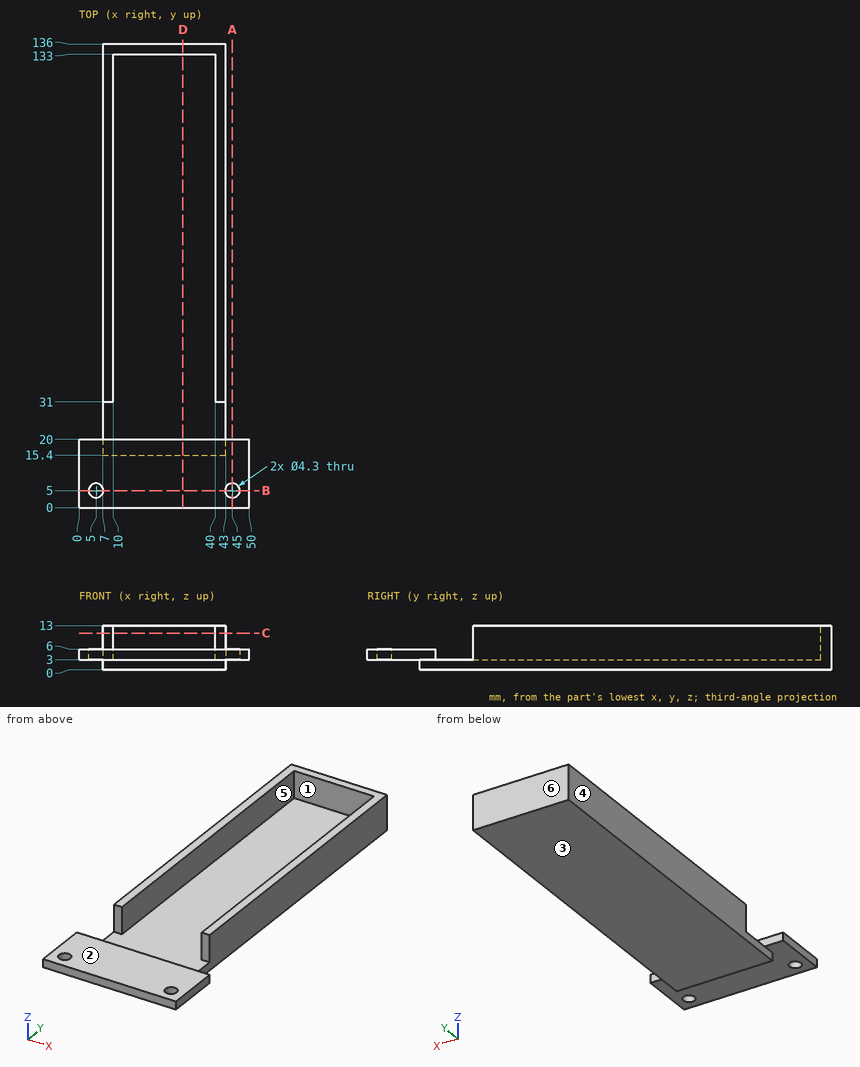
The drawing under review shows one solid part. Ordinate dimensions are in mm from its lowest x, y, z. A direction names the side the tool comes from. Round coordinates to 2 decimals unless told otherwise and drop trailing zeros. Loops run counter-clockwise (first coordinate to the right, second up) from the corner with the lowest first, then second, coordinate; pieces in that order, holes last. Notation, with made-up numbers: (45.25, 76) - (63.25, 76) arc R18 cw to (63.25, 83) - close; hole circle Ø5 at (32.25, 1.25). An arc over 180 degrees is marked (long way). Use a Markdown table: item, result. Add a question column.
Q1. Add section D-D (x = 30.5). State the section outline as (y, z) points, plus the area to 3 significant figures.
Q2. The part is to be moulded in two halves that separate along Y. For the marked faces 4, 5 and 6, say which applies: pulls with the +Y half, pulls with the -Y half, needs draft (parallel to the pull), parting line crosses it, or undercut.
Q3. Insertion check: pin 1 Ø5.5 at (x, y) = (5, 5) entering from +Z; pin 2 Ø1 at (y, z) = (109.5, 7.5) entering from -X; pin 3 Ø3.5 at (x, y) = (45, 5) entering from +Z; pin 4 Ø1.5 at (x, z) = (31, 1.5) entering from -Y. Each pin has a flat end and moves straight along its axis. Give the tip position at first contact, or say it passes through.
Q4. Add section C-C (z = 10.75). State the section outline as (x, y) points.
Q5. Machinability: for the marked faces 1, 2 and 3, which of the approach directions +Z, -Z, +X, -X, +Y, -Y give a long, thin tool a straight path to every point of the face, cutting with its end or side? Answer none if there is none.
Q6. Add section A-A (x = 45). State the section outline as (y, z) points.
Q7. Add section B-B (y = 5). State the section outline as (x, z) points.
Q8. For probe 1 along Y at (x, z) = (45, 4.3); probe 2 along X at (y, z) = (110.5, 8); probe 3 along Y at (x, z) = (35, 3.75), list the stretches that pass through material, from the lowest coordinate up.
Worked answers:
| question | item | result |
|---|---|---|
| 1 | outline | (0, 3) - (15.4, 3) - (15.4, 0) - (136, 0) - (136, 13) - (133, 13) - (133, 3) - (20, 3) - (20, 6) - (0, 6) - close |
| 1 | area | 452 mm² |
| 2 | face 4 | needs draft |
| 2 | face 5 | undercut |
| 2 | face 6 | pulls with the +Y half |
| 3 | pin 1 | z = 6 |
| 3 | pin 2 | x = 7 |
| 3 | pin 3 | through |
| 3 | pin 4 | y = 15.4 |
| 4 | outline | (7, 31) - (10, 31) - (10, 133) - (40, 133) - (40, 31) - (43, 31) - (43, 136) - (7, 136) - close |
| 5 | face 1 | +Z |
| 5 | face 2 | +Z, +X, -X, -Y |
| 5 | face 3 | -Z, +X, -X, +Y, -Y |
| 6 | outline | (0, 3) - (2.85, 3) - (2.85, 6) - (0, 6) - close; (7.15, 3) - (20, 3) - (20, 6) - (7.15, 6) - close |
| 7 | outline | (0, 3) - (2.85, 3) - (2.85, 6) - (0, 6) - close; (7.15, 3) - (42.85, 3) - (42.85, 6) - (7.15, 6) - close; (47.15, 3) - (50, 3) - (50, 6) - (47.15, 6) - close |
| 8 | probe 1 | 0 to 2.85, 7.15 to 20 |
| 8 | probe 2 | 7 to 10, 40 to 43 |
| 8 | probe 3 | 0 to 20, 133 to 136 |
